Geometry check sheet. Reference: the model listing, model coordinates, mm. A direction names the side the tool comes from. Round coordinates to 2 decimals unless told otherwise and drop trailing zeros. Write each loop counter-clockwise with the first axis right and the second up, starting at its lowest first coordinate (ties: lowest second). Pieces come first, ordered by that corner, then holes. Notation, with made-up numbers: M -5.75,24.25 L 43.25,24.25 A19 ccw 43.25,57.25 Z; hole C 42.5,46.5 d8. An arc over 180 degrees is marked long. One line per item, written item: value. Start each with the question number.
1. Section check B-B (y = 17). Record the boundary of the cut face in (x, z), and give its area (3 significant figures).
2. Section check A-A (x = 25.1). Record the boundary of the cut face in (y, z), and give its area (4 significant figures).
3. Release check for a two-part mould opening along Y. For faces 4 (the flat face through (0, 8, 6)), 5 (the flat face through (-2.53, 15.8, 4.66)), 6 (the flat face through (-2.53, 18.3, 4.66)), 7 (the flat face through (-2, 5, 9.1)) record: pulls with the +Y half, pulls with the -Y half, needs draft (parallel to the pull), parting line crosses it, or undercut.
4. Depth check by flat-ended pin: P1, Ø3, axis at x = -2.5, z = 6.1, coming from the -Y side; P2, Ø1.5, axis at x = 25.5, z = 5.5, coming from the +Y side; P3, Ø1, axis at x = 8, y = 22, coming from the -Z side; P4, Ø1.5, axis at y = 11.5, z = 2.5, coming from the -X side. Enter the tip coordinate at first touch or a pass-through.
5. Access from +Z, -Z, +X, -X, +Y, -Y to the whole of each face (thin tool, end or side, straight path). Record for faces 1 (the cylindrical face through (0, 25, 6)), 2 (the flat face through (22.6, 8, 6)), 3 (the flat face through (-2, 4, 3.1)).
6. Section check C-C (z = 4.25). Record the boundary of the cut face in (x, y).
7. Section check D-D (x = 8). Record the boundary of the cut face in (y, z).
8. Scan lines: probe 1 along Z at (x, y) = (-2.5, 17.2); probe 2 along X at (y, z) = (17, 5); probe 3 along Y at (x, z) = (25, 10). Record each from-to range of solid material in increasing order. Write a range as [from, to].
Autodesk Inventor part; units mm, degrees
ref_plane "工作平面1" through (0, 15.8, 0) normal (0, 1, 0) x (1, 0, 0)
ref_plane "YZ Plane" through (0, 0, 0) normal (1, 0, 0) x (0, 1, 0)
ref_plane "XZ Plane" through (0, 0, 0) normal (0, 1, 0) x (-1, 0, 0)
sketch "草图1" plane through (0, 0, 0) normal (0, 1, 0) x (-1, 0, 0)
  line L0 (0, 0) -> (-22.6, 0)
  line L1 (-22.6, 0) -> (-22.6, 12.2)
  line L2 (-22.6, 12.2) -> (0, 12.2)
  line L3 (0, 12.2) -> (0, 0)
  dimension "d0" = 22.6
  dimension "d1" = 12.2
extrude "拉伸1" add sketch "草图1" along normal blind 22.8
ref_plane "工作平面1" through (0, 15.8, 0) normal (0, 1, 0) x (1, 0, 0)
sketch "草图2" plane through (0, 15.8, 0) normal (0, 1, 0) x (1, 0, 0)
  line L0 (-5, -12.2) -> (27.6, -12.2)
  line L1 (27.6, -12.2) -> (27.6, 0)
  line L2 (27.6, 0) -> (-5, 0)
  line L3 (-5, 0) -> (-5, -12.2)
  line L4 (0, -12.2) -> (22.6, -12.2)
  line L5 (22.6, -12.2) -> (22.6, 0)
  line L6 (22.6, 0) -> (0, 0)
  line L7 (0, 0) -> (0, -12.2)
  line L8 (22.6, 0) -> (0, 0)
  line L9 (0, -12.2) -> (22.6, -12.2)
  dimension "d5" = 5
  dimension "d6" = 5
extrude "拉伸2" add sketch "草图2" along normal blind 2.5
sketch "草图3" plane through (0, 22.8, 0) normal (0, 1, 0) x (1, 0, 0)
  line L0 (0, -12.2) -> (22.6, -12.2)
  line L1 (22.6, -12.2) -> (22.6, 0)
  line L2 (22.6, 0) -> (0, 0)
  line L3 (0, 0) -> (0, -12.2)
  circle A0 centre (6.1, -6.1) radius 6.1
  line L4 (0, 0) -> (0, -12.2)
  line L5 (0, -6.1) -> (6.1, -6.1) construction
  circle A1 centre (11.85, -6.1) radius 2.75
  line L6 (14.6, -6.1) -> (0, -6.1) construction
  point P0 (11.553, -3.3661)
  point P1 (11.553, -8.8339)
  dimension "d14" = 5.5
  dimension "d15" = 14.6
extrude "拉伸3" add sketch "草图3" along normal blind 4.4 contours A0 A1 | A1 A0 | A0 A1
sketch "草图4" plane through (6.1, 27.2, 6.1) normal (0, 1, 0) x (0, 0, 1)
  arc A0 (-2.7339, 5.453) -> (2.7339, 5.453) centre (0, 0) ccw
  circle A1 centre (0, 0) radius 2.35
  arc A2 (2.7339, 5.453) -> (-2.7339, 5.453) centre (0, 5.75) ccw
  point P0 (-6.1, -6.1)
  dimension "d16" = 4.7
extrude "拉伸4" add sketch "草图4" along normal blind 3 contours A1
sketch "草图5" plane through (0, 18.3, 0) normal (0, 1, 0) x (1, 0, 0)
  line L0 (0, 0) -> (0, -12.2)
  line L1 (0, 0) -> (-5, 0)
  line L2 (-5, 0) -> (-5, -12.2)
  line L3 (-5, -12.2) -> (0, -12.2)
  line L4 (22.6, -12.2) -> (22.6, 0)
  line L5 (22.6, -12.2) -> (27.6, -12.2)
  line L6 (27.6, -12.2) -> (27.6, 0)
  line L7 (27.6, 0) -> (22.6, 0)
  circle A0 centre (-2.5, -6.1) radius 1.25
  circle A1 centre (25.1, -6.1) radius 1.25
  line L8 (-5, 0) -> (-5, -12.2)
  line L9 (-5, -6.1) -> (-2.5, -6.1) construction
  line L10 (-5, -6.7) -> (-3.5966, -6.7)
  line L11 (-5, -5.5) -> (-3.5966, -5.5)
  line L12 (27.6, -12.2) -> (27.6, 0)
  line L13 (27.6, -6.7) -> (26.1966, -6.7)
  line L14 (27.6, -5.5) -> (26.1966, -5.5)
  point P0 (0, 0)
  dimension "d17" = 2.5
  dimension "d18" = 2.5
  dimension "d19" = 2.5
  dimension "d20" = 2.5
  dimension "d21" = 0.6
  dimension "d22" = 0.6
extrude "拉伸5" cut sketch "草图5" against normal through all contours L11 A0 L10 L2 | A0 | L13 A1 L14 L6 | A1
sketch "草图6" plane through (0, 0, 0) normal (-1, 0, 0) x (0, 0, 1)
  line L0 (3.1, 6) -> (9.1, 6)
  line L1 (9.1, 6) -> (9.1, 3)
  line L2 (9.1, 3) -> (3.1, 3)
  line L3 (3.1, 3) -> (3.1, 6)
  line L4 (12.2, 15.8) -> (0, 15.8)
  line L5 (0, 0) -> (0, 15.8)
  line L6 (0, 0) -> (12.2, 0)
  line L7 (12.2, 0) -> (12.2, 15.8)
  line L8 (6.1, 0) -> (6.1, 6) construction
  dimension "d25" = 6
  dimension "d26" = 3
  dimension "d27" = 6
extrude "拉伸6" add sketch "草图6" along normal blind 5 contours L0 L1 L2 L3
ref_plane "工作平面2" through (6.1, 18.3, 12.2) normal (-1, 0, 0) x (0, 0, 1)
properties part number "sg90"
Result sheet:
1. outline: M -5,0 L 27.6,0 L 27.6,5.5 L 26.2,5.5 A1.25 cw long 26.2,6.7 L 27.6,6.7 L 27.6,12.2 L -5,12.2 L -5,6.7 L -3.6,6.7 A1.25 cw long -3.6,5.5 L -5,5.5 Z
1. area: 385 mm2
2. outline: M 15.8,0 L 18.3,0 L 18.3,4.85 L 15.8,4.85 Z; M 15.8,7.35 L 18.3,7.35 L 18.3,12.2 L 15.8,12.2 Z
2. area: 24.25 mm2
3. face 4: undercut
3. face 5: undercut
3. face 6: pulls with the +Y half
3. face 7: needs draft
4. P1: stops at y = 3
4. P2: stops at y = 18.3
4. P3: stops at z = 0
4. P4: stops at x = 0
5. face 1: +Y
5. face 2: +Z, -Z, +X, -Y
5. face 3: -Z, -X, -Y
6. outline: M -5,3 L 0,3 L 0,0 L 22.6,0 L 22.6,15.8 L 27.6,15.8 L 27.6,18.3 L 22.6,18.3 L 22.6,22.8 L 13.88,22.8 L 13.88,27.2 L 7.55,27.2 L 7.55,30.2 L 4.65,30.2 L 4.65,27.2 L 0.29,27.2 L 0.29,22.8 L 0,22.8 L 0,18.3 L -5,18.3 L -5,15.8 L 0,15.8 L 0,6 L -5,6 Z
7. outline: M 0,0 L 22.8,0 L 22.8,0.3 L 27.2,0.3 L 27.2,4.72 L 30.2,4.72 L 30.2,7.48 L 27.2,7.48 L 27.2,11.9 L 22.8,11.9 L 22.8,12.2 L 0,12.2 Z
8. probe 1: z = [0, 4.85], [7.35, 12.2]
8. probe 2: x = [-5, -3.09], [-1.91, 24.51], [25.69, 27.6]
8. probe 3: y = [15.8, 18.3]
